from build123d import *

# Parameters (mm, degrees)
F0_W     = 220
F0_H     = 650
F1_DEPTH = 30
F2_W     = 175
F2_H     = 600
F3_DEPTH = 8
F4_W     = 15
F4_H     = 650
F5_DEPTH = 10


with BuildPart() as f1:
    # F0 (on Front) → F1 (new body)
    with BuildSketch(Plane.XZ):
        with Locations((110, 325)):
            Rectangle(F0_W, F0_H)
    extrude(amount=F1_DEPTH)

    # F2 (on face) → F3 (cut)
    with BuildSketch(Plane.XZ.offset(30)):
        with Locations((117.5, 320)):
            Rectangle(F2_W, F2_H)
    extrude(amount=-F3_DEPTH, mode=Mode.SUBTRACT)

    # F4 (on face) → F5 (join)
    with BuildSketch(Plane.XZ):
        with Locations((7.5, 325)):
            Rectangle(F4_W, F4_H)
    extrude(amount=-F5_DEPTH)


solid = f1.part
Verification items for the finished model (mm, model axes). A direction names the side the tool comes from. Give positions to 0.01 mm unless a question says otherwise; leave off trailing zeros. Write each loop counter-clockwise with the first axis right and the second up, starting at its lowest first coordinate (ties: lowest second). Pieces come first, ordered by that corner, then holes. Notation, with made-up numbers: M 18,39 L 41,39 A21 ccw 41,59 Z; hole C 73,0.25 d9. An arc over 180 degrees is marked long. Put each result on its own line as item: value. Start each with the question number.
1. Set-up check for faces 5 (the face through (116, 0, 330)), 6 (the face through (108, -15, 650)): record each of +Z, -Z, +X, -X, +Y, -Y from which the full face is reachable in a straight line by a thin tool's end or side.
2. Scan lines: line 1 along Z through (x, y) = (200, -28); line 2 along X through (y, z) = (-25, 100.5); line 3 along Y through (x, z) = (40.5, 331). Record each from-to range of solid material in increasing order. Write a range as [from, to].
3. Section check A-A (z = 552.5). Record the cut outline in (x, y), and give its area (3 significant figures).
4. Section check C-C (x = 21.5). Record the cut outline in (y, z).
5. Go/stop test with flat-tipped pins: pin 1 Ø1.5 at (x, z) = (140, 425) entering from +Y; pin 2 Ø1.5 at (x, z) = (152.5, 447) entering from -Y; pin 3 Ø5 at (y, z) = (7, 316) entering from +X. Record where each tip stops, or that it passes through.
6. Draft check along X on faces 1 (the face through (116, -22, 324)), 2 (the face through (0, -10, 320)), 3 (the face through (108, -15, 0)), 4 (the face through (220, -15, 320)). Enter one of: +X half, -X half, draft (parallel to the pull), parting line (faces both ways), or undercut.
7. Section check B-B (x = 85). Record the cut outline in (y, z), and give its area (3 significant figures).
Answer list:
1. face 5: +Z, -Z, +X, +Y
1. face 6: +Z, +X, -X, +Y, -Y
2. line 1: [0, 20], [620, 650]
2. line 2: [0, 30], [205, 220]
2. line 3: [-22, 0]
3. outline: M 0,-30 L 30,-30 L 30,-22 L 205,-22 L 205,-30 L 220,-30 L 220,0 L 15,0 L 15,10 L 0,10 Z
3. area: 5,350 mm2
4. outline: M -30,0 L 0,0 L 0,650 L -30,650 Z
5. pin 1: y = 0
5. pin 2: y = -22
5. pin 3: x = 15
6. face 1: undercut
6. face 2: -X half
6. face 3: draft
6. face 4: +X half
7. outline: M -30,0 L 0,0 L 0,650 L -30,650 L -30,620 L -22,620 L -22,20 L -30,20 Z
7. area: 14,700 mm2
